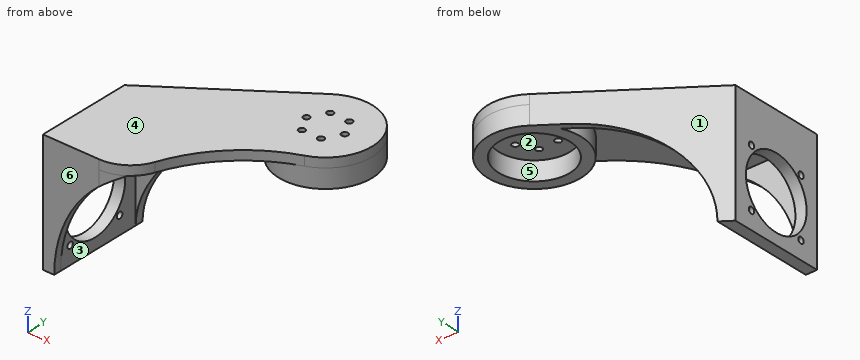
from build123d import *

# Parameters (mm, degrees)
SKIZZE1_R                        = 1.7
AUFSATZ_LINEAR_AUSTRAGEN1_DEPTH  = 5
SKIZZE14_R                       = 25
SKIZZE14_R_2                     = 19
AUFSATZ_LINEAR_AUSTRAGEN9_DEPTH  = 10
SKIZZE4_W                        = 59.5
SKIZZE4_H                        = 51
SKIZZE4_R                        = 1.7
SKIZZE4_R_2                      = 19
AUFSATZ_LINEAR_AUSTRAGEN4_DEPTH  = 6
AUFSATZ_LINEAR_START             = -64.5
AUFSATZ_LINEAR_AUSTRAGEN10_DEPTH = 59.5
AUFSATZ_LINEAR_AUSTRAGEN11_DEPTH = 59.5
SCHNITT_LINEAR_AUSTRAGEN4_DEPTH  = 146.774654862
SKIZZE19_R                       = 67.170138889
SCHNITT_LINEAR_AUSTRAGEN5_DEPTH  = 146.774654862


# Read off the part's stored shape, not the designer's step: Aufsatz-Linear austragen10
with BuildPart() as part:
    # Skizze1 → Aufsatz-Linear austragen1 (new body)
    with BuildSketch(Plane.XY):
        with BuildLine():
            Line((-83, -29), (-83, -80))
            Line((-83, -80), (-53, -80))
            ThreePointArc((-53, -80), (-41.528471273, -76.383040886), (-34.206147584, -66.840402867))
            ThreePointArc((-34.206147584, -66.840402867), (-17.465018587, -40.413653136), (8.789632026, -23.403896446))
            ThreePointArc((8.789632026, -23.403896446), (22.036349892, 11.806747369), (-14.616570826, 20.281909606))
            Line((-14.616570826, 20.281909606), (-83, -29))
        make_face()
        with Locations((10.25, 0)):
            Circle(SKIZZE1_R, mode=Mode.SUBTRACT)
        with Locations((5.125, -8.876760389)):
            Circle(SKIZZE1_R, mode=Mode.SUBTRACT)
        with Locations((-5.125, -8.876760389)):
            Circle(SKIZZE1_R, mode=Mode.SUBTRACT)
        with Locations((-10.25, 0)):
            Circle(SKIZZE1_R, mode=Mode.SUBTRACT)
        with Locations((-5.125, 8.876760389)):
            Circle(SKIZZE1_R, mode=Mode.SUBTRACT)
        with Locations((5.125, 8.876760389)):
            Circle(SKIZZE1_R, mode=Mode.SUBTRACT)
    extrude(amount=-AUFSATZ_LINEAR_AUSTRAGEN1_DEPTH)

    # Skizze14 → Aufsatz-Linear austragen9 (add)
    with BuildSketch(Plane(origin=(0, 0, -5), x_dir=(-1, 0, 0), z_dir=(0, 0, -1))):
        with Locations(Location((0, 0, 0), (0, 0, 249.415691324))):
            Circle(SKIZZE14_R)
        Circle(SKIZZE14_R_2, mode=Mode.SUBTRACT)
    extrude(amount=AUFSATZ_LINEAR_AUSTRAGEN9_DEPTH)

    # Skizze4 → Aufsatz-Linear austragen4 (add)
    with BuildSketch(Plane.ZY.offset(83)):
        with Locations((-34.75, -54.5)):
            Rectangle(SKIZZE4_W, SKIZZE4_H)
        with Locations((-24, -39)):
            Circle(SKIZZE4_R, mode=Mode.SUBTRACT)
        with Locations((-55, -39)):
            Circle(SKIZZE4_R, mode=Mode.SUBTRACT)
        with Locations((-55, -70)):
            Circle(SKIZZE4_R, mode=Mode.SUBTRACT)
        with Locations((-24, -70)):
            Circle(SKIZZE4_R, mode=Mode.SUBTRACT)
        with Locations((-39.5, -54.5)):
            Circle(SKIZZE4_R_2, mode=Mode.SUBTRACT)
    extrude(amount=-AUFSATZ_LINEAR_AUSTRAGEN4_DEPTH)

    # Aufsatz-Linear austragen10 outline → Aufsatz-Linear austragen10 (add)
    with BuildSketch(Plane.XY.offset(AUFSATZ_LINEAR_START)):
        with BuildLine():
            Line((-77, -76), (-77, -80))
            Line((-77, -80), (-53, -80))
            ThreePointArc((-53, -80), (-46.67544468, -78.973665961), (-41, -76))
            Line((-41, -76), (-77, -76))
        make_face()
    extrude(amount=AUFSATZ_LINEAR_AUSTRAGEN10_DEPTH)

    # Skizze16 → Aufsatz-Linear austragen11 (add)
    with BuildSketch(Plane(origin=(0, 0, -5), x_dir=(-1, 0, 0), z_dir=(0, 0, -1))):
        Polygon((83, -29), (14.616570826, 20.281909606), (12.565587056, 17.435970711), (77, -29), align=None)
    extrude(amount=AUFSATZ_LINEAR_AUSTRAGEN11_DEPTH)

    # Skizze18 → Schnitt-Linear austragen4 (cut, through all)
    with BuildSketch(Plane(origin=(0, -76, 0), x_dir=(1, 0, 0), z_dir=(0, 1, 0))):
        with BuildLine():
            Line((25, 15), (25, 103.581922368))
            Line((25, 103.581922368), (-57.878501345, 103.581922368))
            ThreePointArc((-57.878501345, 103.581922368), (-74.323098772, 48.442371863), (-27.5, 15))
            Line((-27.5, 15), (25, 15))
        make_face()
    extrude(amount=SCHNITT_LINEAR_AUSTRAGEN4_DEPTH, mode=Mode.SUBTRACT)

    # Skizze19 → Schnitt-Linear austragen5 (cut, through all)
    with BuildSketch(Plane(origin=(0, -76, 0), x_dir=(1, 0, 0), z_dir=(0, 1, 0))):
        with Locations((-9.829861111, 64.5)):
            Circle(SKIZZE19_R)
    extrude(amount=-SCHNITT_LINEAR_AUSTRAGEN5_DEPTH, mode=Mode.SUBTRACT)


solid = part.part
The listing builds one solid part. Answer for the finished solid, in the listing's coordinates (mm). Face numbers are marked on the shaded views. A direction names the side the tool comes from. Round coordinates to 2 decimals unless told otherwise and drop trailing zeros. Order: outer loops, then holes, each group sorted by start corner. A loop starts at its lowest first (then second) coordinate and runs counter-clockwise, first axis right, second up. Notation, with made-up numbers: (-5, 2.25) -> (41, 2.25) arc R18 ccw to (41, 11.25) -> close; hole circle Ø10 at (-30.75, -30). An arc over 180 degrees is marked (long way). One line per item, written item: value.
Item 1: Given P1, Ø4, axis at y = -10, z = -23.5, coming from the +X side; P2, Ø12, axis at x = -46, y = -9, coming from the -Z side; P3, Ø10, axis at x = 13.5, y = -0.5, coming from the -Z side, each flat-ended and moving along its own axis, determine where each tip first touches the part or whether it passes through.
Taken from the geometry:
P1: stops at x = -52.02
P2: stops at z = -21.49
P3: stops at z = -5
Item 2: Find section C-C, the plane y = 0. Give the vertices of the cut face in (x, z), then the cut area to 3 significant figures.
Taken from the geometry:
outline: (-42.76, -17.41) arc R49.5 cw to (-36.76, -15.87) -> (-36.76, -5) -> (-25, -5) -> (-25, -15) -> (-19, -15) -> (-19, -5) -> (-11.95, -5) -> (-11.95, 0) -> (-42.76, 0) -> close; (-8.55, -5) -> (8.55, -5) -> (8.55, 0) -> (-8.55, 0) -> close; (11.95, -5) -> (19, -5) -> (19, -15) -> (25, -15) -> (25, 0) -> (11.95, 0) -> close
area: 494 mm2
Item 3: For the marked faces 1, 2 and 3, determine the directions among +Z, -Z, +X, -X, +Y, -Y from which every point of the face is accessible in a straight line to the end or side of a thin tool.
Taken from the geometry:
face 1: +Z, -Z, -X, +Y
face 2: -Z
face 3: -Z, +X
Item 4: For a pull along Y with two mould halves and no side action, classify the marked faces 4, 5 and 6 as released by +Y, released by -Y, zero draft, split by the parting line, or undercut.
Taken from the geometry:
face 4: zero draft
face 5: undercut
face 6: released by -Y
Item 5: Find section D-D, the plane z = -11. Give the vertices of the cut face in (x, y).
Taken from the geometry:
outline: (-83, -80) -> (-53, -80) arc R20 ccw to (-50.44, -79.84) -> (-50.44, -76) -> (-77, -76) -> (-77, -29) -> (-22.93, 9.97) arc R25 ccw (long way) to (-14.62, 20.28) -> (-83, -29) -> close; hole circle Ø38 at (0, 0)
Item 6: Find section A-A, the plane y = -39. Give the vertices of the cut face in (x, z), then the cut area to 3 significant figures.
Taken from the geometry:
outline: (-83, -64.5) -> (-77, -64.5) -> (-77, -56.7) -> (-83, -56.7) -> close; (-83, -53.3) -> (-77, -53.3) -> (-77, -50.49) -> (-83, -50.49) -> close; (-83, -28.51) -> (-77, -28.51) -> (-77, -25.7) -> (-83, -25.7) -> close; (-83, -22.3) -> (-77, -22.3) -> (-77, -5) -> (-16.03, -5) -> (-16.03, 0) -> (-83, 0) -> close
area: 519 mm2
Item 7: Straight lines are drawn through the part: L1, parallel to Z at x = -78, y = -70; L2, parallel to Z at x = -79, y = -54; L3, parallel to X at y = -11.5, z = -14. For each, find the intervals that lie inside material, in ascending order.
Taken from the geometry:
L1: z = -64.5 to -56.7, -53.3 to -50.49, -28.51 to -25.7, -22.3 to 0
L2: z = -64.5 to -58.49, -20.51 to 0
L3: x = -58.72 to -52.72, -22.2 to -15.12, 15.12 to 22.2
Item 8: Find section B-B, the plane x = -10.25. Give the vertices of the cut face in (y, z).
Taken from the geometry:
outline: (-34.03, -5) -> (-22.8, -5) -> (-22.8, -15) -> (-16, -15) -> (-16, -5) -> (-1.7, -5) -> (-1.7, 0) -> (-34.03, 0) -> close; (1.7, -5) -> (16, -5) -> (16, -15) -> (22.8, -15) -> (22.8, 0) -> (1.7, 0) -> close
